```python
from build123d import *

# Parameters (mm, degrees)
SKETCH1_R                     = 23.5
BOSS_EXTRUDE1_DEPTH           = 5.12
SKETCH2_R                     = 17.5
BOSS_EXTRUDE2_DEPTH           = 7
SKETCH3_R                     = 9
BOSS_EXTRUDE3_DEPTH           = 13
CSK_FOR_M5_SFHCS1_D           = 5.3
CSK_FOR_M5_SFHCS1_CSINK_D     = 11.2
CSK_FOR_M5_SFHCS1_CSINK_ANGLE = 90


with BuildPart() as part:
    # Sketch1 → Boss-Extrude1 (new body)
    with BuildSketch(Plane.XY):
        Circle(SKETCH1_R)
    extrude(amount=BOSS_EXTRUDE1_DEPTH)

    # Sketch2 → Boss-Extrude2 (add)
    with BuildSketch(Plane.XY.offset(5.12)):
        Circle(SKETCH2_R)
    extrude(amount=BOSS_EXTRUDE2_DEPTH)

    # Sketch3 → Boss-Extrude3 (add)
    with BuildSketch(Plane.XY.offset(12.12)):
        Circle(SKETCH3_R)
    extrude(amount=BOSS_EXTRUDE3_DEPTH)

    # CSK for M5 SFHCS1 (through all)
    with Locations(Plane(origin=(0, 0, 0), x_dir=(-1, 0, 0), z_dir=(0, 0, -1))):
        with Locations((0, 0)):
            CounterSinkHole(CSK_FOR_M5_SFHCS1_D / 2, CSK_FOR_M5_SFHCS1_CSINK_D / 2, counter_sink_angle=CSK_FOR_M5_SFHCS1_CSINK_ANGLE)


solid = part.part
```
Read the model definition and answer for the solid it produces. Units are mm, in the model's axes. A direction names the side the tool comes from. Coordinates: 2 decimals unless noted, no trailing zeros. Loops run counter-clockwise (first coordinate to the right, second up) from the corner with the lowest first, then second, coordinate; pieces in that order, holes last.
(1) The part is cut by section C-C (z = 22). Determine the outline of the cut face in (x, y).
Solution:
outline: circle Ø18 at (0, 0); hole circle Ø5.3 at (0, 0)
(2) Consider line 1 along Y through (x, z) = (0, 12); line 2 along Y through (x, z) = (0, 14.5); line 3 along Z through (x, y) = (7.5, 16.5). Determine where each line is inside the solid, lowest interval first.
Solution:
line 1: y = -17.5 to -2.65, 2.65 to 17.5
line 2: y = -9 to -2.65, 2.65 to 9
line 3: z = 0 to 5.12
(3) The part is cut by section A-A (x = 0). Determine the outline of the cut face in (y, z).
Solution:
outline: (-23.5, 0) - (-5.6, 0) - (-2.65, 2.95) - (-2.65, 25.12) - (-9, 25.12) - (-9, 12.12) - (-17.5, 12.12) - (-17.5, 5.12) - (-23.5, 5.12) - close; (2.65, 2.95) - (5.6, 0) - (23.5, 0) - (23.5, 5.12) - (17.5, 5.12) - (17.5, 12.12) - (9, 12.12) - (9, 25.12) - (2.65, 25.12) - close
(4) A tool of negligible diameter and unlimited length cuts with its end or side. For faces 4 (the face through (2.45, -1.01, 14.19)), 5 (the face through (0, 18, 5.12)), from which of +Z, -Z, +X, -X, +Y, -Y can it reach the whole face along a straight path? Write none if from no direction.
Solution:
face 4: +Z, -Z
face 5: +Z
(5) The part is cut by section D-D (y = 15). Determine the outline of the cut face in (x, z), and give its area (3 significant figures).
Solution:
outline: (-18.09, 0) - (18.09, 0) - (18.09, 5.12) - (9.01, 5.12) - (9.01, 12.12) - (-9.01, 12.12) - (-9.01, 5.12) - (-18.09, 5.12) - close
area: 311 mm2
(6) The mould has two halves that part along X. Classify faces 1 (the face through (-0.364, 2.769, 2.807)), 2 (the face through (5, -5, 0)), 3 (the face through (-1.172, 8.923, 18.529)): released by +X, released by -X, zero draft, split by the parting line, or undercut.
Solution:
face 1: undercut
face 2: zero draft
face 3: split by the parting line
(7) Flat-ended cylindrical pins translate along their axes: pin 1 Ø6 at (y, z) = (13.5, 10) entering from -X; pin 2 Ø8 at (y, z) = (-15, 6) entering from -X; pin 3 Ø12 at (y, z) = (-16.5, 7) entering from +X. Find the tip coordinate at first contact, or state that the pin passes through.
Solution:
pin 1: stops at x = -14
pin 2: stops at x = -20.71
pin 3: stops at x = 20.87
